Input: part model. Units: mm. Frame: model coordinates. A direction names the side the tool comes from. Give positions to 0.01 mm unless a question says otherwise; leave off trailing zeros. Write each loop counter-clockwise with the first axis right and the second up, starting at its lowest first coordinate (ties: lowest second). Pieces come first, ordered by that corner, then holes. Notation, with made-up numbers: (8.25, 33.5) -> (33.25, 33.5) arc R16 ccw to (33.25, 42.5) -> close; hole circle Ø1 at (87.25, 31.25). An arc over 180 degrees is marked (long way). Return JSON: item names as keys, results as strings. Group by question number.
Item 1: Section C-C, the plane z = -17. Return loops of the section in (x, y).
Item 2: Set-up query: faces 1 (the face through (-42, 0, -3.175)), 2 (the face through (0, -4.762, -37)). Return all of +Z, -Z, +X, -X, +Y, -Y with unobstructed straight access to the full face (end or side cutting, diameter ignored); none if empty.
Item 3: Pin query (flat end, axial travel): P1, Ø1, axis at x = 26, y = 1.5, coming from the +Z side; P2, Ø5, axis at y = 3, z = -9.5, coming from the +X side; P3, Ø2, axis at y = 2.5, z = -29, coming from the +X side. Return the tip coordinate at first contact, or that it passes through.
Item 4: Section A-A, the plane z = -30.5. Return loops of the section in (x, y), then the cut area to 3 significant figures.
Item 5: Section B-B, the plane y = -2.5. Return loops of the section in (x, z) (3 decimals), then the cut area to 3 significant figures.
Item 6: Section D-D, the plane x = -4. Return loops of the section in (y, z), then the cut area to 3 significant figures.
Item 7: Line query: line 1 (X direction, y = -2.75, z = -31.5); line 2 (X direction, y = -0.5, z = -11.5); line 3 (Z direction, x = 4, y = 2.75). Output: solid intervals per line, ascending. Write a range as [from, to].
Item 8: Mould query, pull axis X, two halves, no side actions, for faces 3 (the face through (45.72, 0, -2)), 4 (the face through (-45.72, 0, -2)), 5 (the face through (0.796, 0.067, -36.186)), 6 (the face through (42, 0, -3.175)). Classes: released by +X, released by -X, zero draft, split by the parting line, or undercut.
from build123d import *

# Parameters (mm, degrees)
SKETCH1_W           = 3.175
SKETCH1_H           = 9.525
REVOLVE1_ANGLE      = 180
BOSS_EXTRUDE1_REACH = 80.74
SKETCH2_W           = 3.175
SKETCH2_H           = 9.525
SKETCH2_2_W         = 3.175
SKETCH2_2_H         = 9.525
BOSS_EXTRUDE2_DEPTH = 6.35
BOSS_EXTRUDE3_REACH = 87.09
SKETCH4_W           = 3.175
SKETCH4_H           = 9.525
SKETCH4_2_W         = 3.175
SKETCH4_2_H         = 9.525
BOSS_EXTRUDE4_DEPTH = 6.35


with BuildPart() as part:
    # Sketch1 → Revolve1 (revolve)
    with BuildSketch(Plane.XY):
        with Locations((37.7825, 0)):
            Rectangle(SKETCH1_W, SKETCH1_H)
    revolve(axis=Axis((0, -72.106361407, 0), (0, 1, 0)), revolution_arc=REVOLVE1_ANGLE)

    # Sketch2 → Boss-Extrude1 (add, up to next)
    with BuildSketch(Plane(origin=(39.37, 0, 0), x_dir=(0, 0, -1), z_dir=(1, 0, 0)), mode=Mode.PRIVATE) as boss_extrude1_sk1:
        with Locations((1.5875, 0)):
            Rectangle(SKETCH2_W, SKETCH2_H)
    boss_extrude1_tool1 = extrude(boss_extrude1_sk1.sketch, amount=-BOSS_EXTRUDE1_REACH, mode=Mode.PRIVATE) - part.part
    add(boss_extrude1_tool1.solids().sort_by_distance((39.37, 0, -1.5875))[0])

    # Sketch2_2 → Boss-Extrude2 (add)
    with BuildSketch(Plane(origin=(39.37, 0, 0), x_dir=(0, 0, -1), z_dir=(1, 0, 0))):
        with Locations((1.5875, 0)):
            Rectangle(SKETCH2_2_W, SKETCH2_2_H)
    extrude(amount=BOSS_EXTRUDE2_DEPTH)

    # Sketch4 → Boss-Extrude3 (add, up to next)
    with BuildSketch(Plane.ZY.offset(39.37), mode=Mode.PRIVATE) as boss_extrude3_sk1:
        with Locations((-1.5875, 0)):
            Rectangle(SKETCH4_W, SKETCH4_H)
    boss_extrude3_tool1 = extrude(boss_extrude3_sk1.sketch, amount=-BOSS_EXTRUDE3_REACH, mode=Mode.PRIVATE) - part.part
    add(boss_extrude3_tool1.solids().sort_by_distance((-39.37, 0, -1.5875))[0])

    # Sketch4_2 → Boss-Extrude4 (add)
    with BuildSketch(Plane.ZY.offset(39.37)):
        with Locations((-1.5875, 0)):
            Rectangle(SKETCH4_2_W, SKETCH4_2_H)
    extrude(amount=BOSS_EXTRUDE4_DEPTH)


solid = part.part
Answer below:
{
 "1": {"outline": "(-35.51, -4.76) -> (-31.95, -4.76) -> (-31.95, 4.76) -> (-35.51, 4.76) -> close; (31.95, -4.76) -> (35.51, -4.76) -> (35.51, 4.76) -> (31.95, 4.76) -> close"},
 "2": {"face 1": "-Z, -X, +Y, -Y", "face 2": "+Z, -Z, +X, -X, -Y"},
 "3": {"P1": "stops at z = -24.65", "P2": "stops at x = 38.74", "P3": "stops at x = 27.68"},
 "4": {"outline": "(-24.89, -4.76) -> (-19.49, -4.76) -> (-19.49, 4.76) -> (-24.89, 4.76) -> close; (19.49, -4.76) -> (24.89, -4.76) -> (24.89, 4.76) -> (19.49, 4.76) -> close", "area": "103 mm2"},
 "5": {"outline": "(-45.72, -3.175) -> (-39.242, -3.175) arc R39.37 ccw to (39.242, -3.175) -> (45.72, -3.175) -> (45.72, 0) -> (36.195, 0) arc R36.195 cw to (-36.195, 0) -> (-45.72, 0) -> close", "area": "417 mm2"},
 "6": {"outline": "(-4.76, -39.17) -> (4.76, -39.17) -> (4.76, -35.97) -> (-4.76, -35.97) -> close", "area": "30.4 mm2"},
 "7": {"line 1": "x = [-23.62, -17.83], [17.83, 23.62]", "line 2": "x = [-37.65, -34.32], [34.32, 37.65]", "line 3": "z = [-39.17, -35.97]"},
 "8": {"face 3": "released by +X", "face 4": "released by -X", "face 5": "undercut", "face 6": "zero draft"}
}
